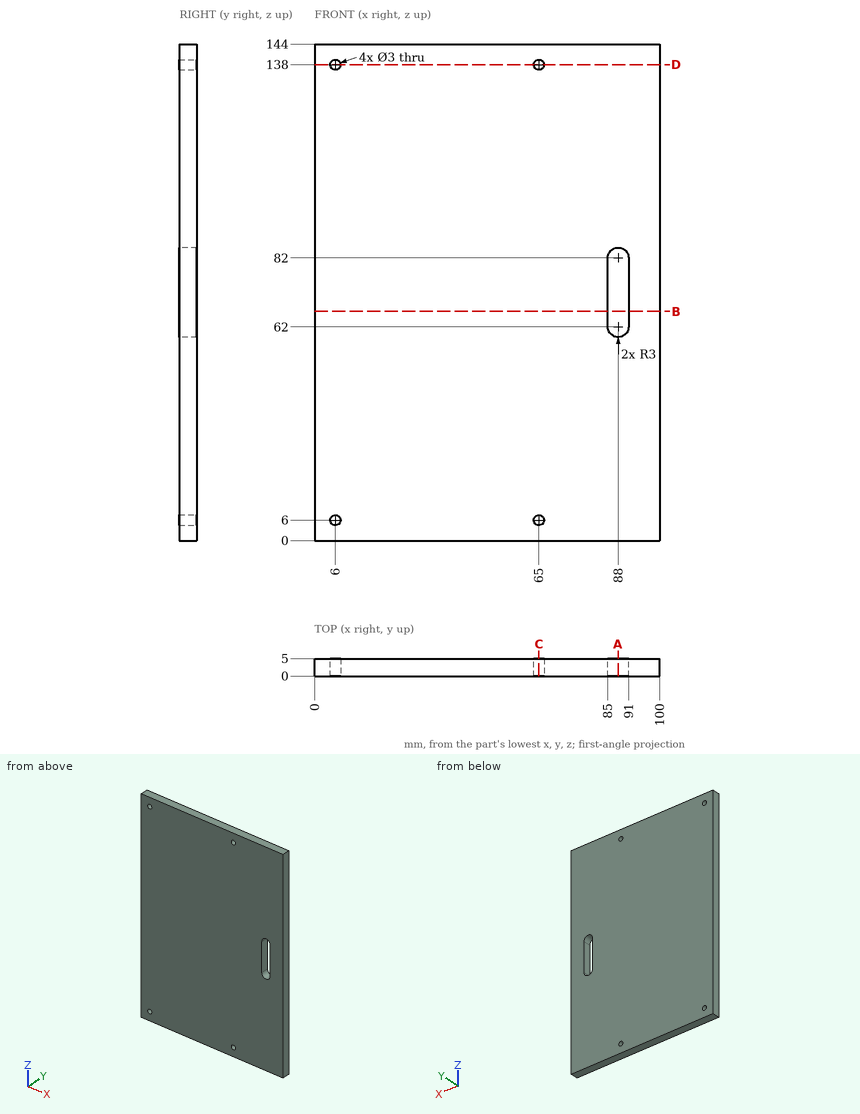
Could you check a few things on this drawing? It's one solid part, dimensions in mm from its lowest x, y, z. Coordinates: 2 decimals unless noted, no trailing zeros. Order: outer loops, then holes, each group sorted by start corner. A loop starts at its lowest first (then second) coordinate and runs counter-clockwise, first axis right, second up.
1) Imagine slicing it at B-B on z = 66.5. List the corners of the cut face in (x, y) for me, and give its area (3 significant figures).
2) Imagine slicing it at A-A on x = 88. List the corners of the cut face in (y, z) for me.
3) I need wall thicknesses on line 1 (Z direction, x = 6, y = 3.35); line 2 (X direction, y = 1.85, z = 138); line 3 (X direction, y = 1.1, z = 77). Which ranges of each line are inside material? Lowest first, please.
4) Imagine slicing it at D-D on z = 138. List the corners of the cut face in (x, y) for me, and give its area (3 significant figures).
5) Imagine slicing it at C-C on x = 65. List the corners of the cut face in (y, z) for me, and give its area (3 significant figures).
Response values:
1. outline: (0, 0) - (85, 0) - (85, 5) - (0, 5) - close; (91, 0) - (100, 0) - (100, 5) - (91, 5) - close
1. area: 470 mm2
2. outline: (0, 0) - (5, 0) - (5, 59) - (0, 59) - close; (0, 85) - (5, 85) - (5, 144) - (0, 144) - close
3. line 1: z = 0 to 4.5, 7.5 to 136.5, 139.5 to 144
3. line 2: x = 0 to 4.5, 7.5 to 63.5, 66.5 to 100
3. line 3: x = 0 to 85, 91 to 100
4. outline: (0, 0) - (4.5, 0) - (4.5, 5) - (0, 5) - close; (7.5, 0) - (63.5, 0) - (63.5, 5) - (7.5, 5) - close; (66.5, 0) - (100, 0) - (100, 5) - (66.5, 5) - close
4. area: 470 mm2
5. outline: (0, 0) - (5, 0) - (5, 4.5) - (0, 4.5) - close; (0, 7.5) - (5, 7.5) - (5, 136.5) - (0, 136.5) - close; (0, 139.5) - (5, 139.5) - (5, 144) - (0, 144) - close
5. area: 690 mm2
